Input: part model. Units: mm. Frame: model coordinates. Face numbers are marked on the shaded views. A direction names the side the tool comes from. Give positions to 0.01 mm unless a question says otherwise; leave off trailing zeros. Loops run counter-clockwise (first coordinate to the right, second up) from the corner with the lowest first, then second, coordinate; pieces in that order, holes last. Notation, with made-up numbers: (85.25, 21.5) -> (102.25, 21.5) arc R12 cw to (102.25, 41.5) -> close; hole circle Ø2 at (43.25, 53.5). An arc over 180 degrees is marked (long way). Use CSV: the item, a comma, the result in double quotes.
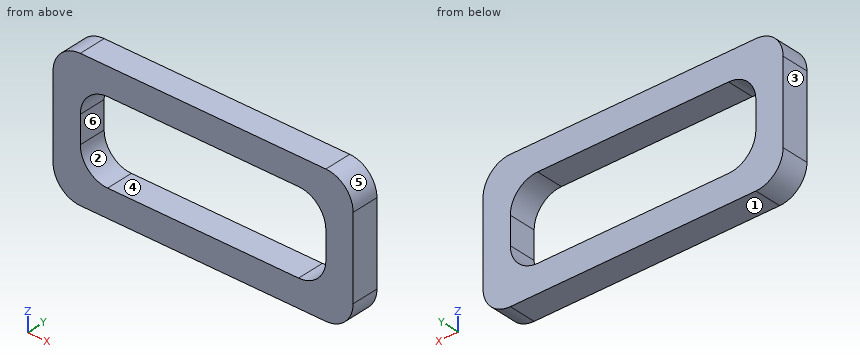
```python
from build123d import *

# Parameters (mm, degrees)
SKETCH3_W = 5
SKETCH3_H = 5
FILLET1_R = 5


with BuildPart() as part:
    # Sweep2: sweep along a path in Sketch4
    with BuildLine(Plane(origin=(0, 0, 0), x_dir=(1, 0, 0), z_dir=(0, 1, 0))) as sweep2_path:
        Line((0, 0), (50, 0))
        Line((50, 0), (50, -20))
        Line((50, -20), (0, -20))
        Line((0, -20), (0, 0))
    # Sketch3 → Sweep2 (sweep)
    with BuildSketch(Plane(origin=(0, 0, 0), x_dir=(0, 0, -1), z_dir=(1, 0, 0))):
        Rectangle(SKETCH3_W, SKETCH3_H)
    sweep(path=sweep2_path.line, transition=Transition.RIGHT)

    # Fillet1
    fillet1_edges = [part.edges().sort_by_distance(p)[0] for p in [
        (-2.5, 0, 22.5),
        (2.5, 0, 17.5),
        (47.5, 0, 2.5),
        (52.5, 0, -2.5),
        (-2.5, 0, -2.5),
        (2.5, 0, 2.5),
        (52.5, 0, 22.5),
        (47.5, 0, 17.5),
    ]]
    fillet(fillet1_edges, radius=FILLET1_R)


solid = part.part
```
1) Section query B-B (y = -1.95). Return loops of the section in (x, z).
From the geometry:
outline,"(-2.5, 2.5) arc R5 ccw to (2.5, -2.5) -> (47.5, -2.5) arc R5 ccw to (52.5, 2.5) -> (52.5, 17.5) arc R5 ccw to (47.5, 22.5) -> (2.5, 22.5) arc R5 ccw to (-2.5, 17.5) -> close; hole (2.5, 7.5) arc R5 ccw to (7.5, 2.5) -> (42.5, 2.5) arc R5 ccw to (47.5, 7.5) -> (47.5, 12.5) arc R5 ccw to (42.5, 17.5) -> (7.5, 17.5) arc R5 ccw to (2.5, 12.5) -> close"
2) Ray query, line 1 (X direction, y = -0.55, z = 8.25); line 2 (Z direction, x = 19.5, y = -1.7); line 3 (X direction, y = -0.55, z = 16). Return the intervals inside material, ascending.
From the geometry:
line 1,"x = -2.5 to 2.5, 47.5 to 52.5"
line 2,"z = -2.5 to 2.5, 17.5 to 22.5"
line 3,"x = -2.5 to 3.93, 46.07 to 52.5"
3) Reachability of the marked faces 5 and 6 from +Z, -Z, +X, -X, +Y, -Y: full face, straight path, thin tool, end or side. Return the list, or none.
From the geometry:
face 5,"+Z, +X, +Y, -Y"
face 6,"+Y, -Y"
4) Section query C-C (x = 18). Return loops of the section in (y, z), then the cut area to 3 significant figures.
From the geometry:
outline,"(-2.5, -2.5) -> (2.5, -2.5) -> (2.5, 2.5) -> (-2.5, 2.5) -> close; (-2.5, 17.5) -> (2.5, 17.5) -> (2.5, 22.5) -> (-2.5, 22.5) -> close"
area,"50.0 mm^2"
5) Mould query, pull axis X, two halves, no side actions, for the marked faces 1, 2, 3 and 4. Classes: pulls with the +X half, pulls with the -X half, needs draft (parallel to the pull), parting line crosses it, or undercut.
From the geometry:
face 1,"needs draft"
face 2,"undercut"
face 3,"pulls with the -X half"
face 4,"undercut"
6) Section query A-A (z = 11.75). Return loops of the section in (x, y).
From the geometry:
outline,"(-2.5, -2.5) -> (2.5, -2.5) -> (2.5, 2.5) -> (-2.5, 2.5) -> close; (47.5, -2.5) -> (52.5, -2.5) -> (52.5, 2.5) -> (47.5, 2.5) -> close"
